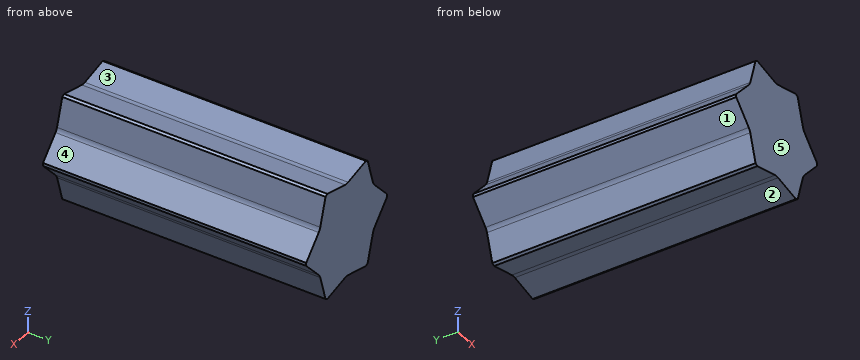
from build123d import *

# Parameters (mm, degrees)
EXTRUDE_1_DEPTH     = 1500
CUT_EXTRUDE_4_DEPTH = 1500
SHELL_START         = 10
SHELL_3_DEPTH       = 1480


# Read off the part's stored shape, not the designer's step: 抽壳3
with BuildPart() as part:
    # 草图2 → 凸台-拉伸1 (new body)
    with BuildSketch(Plane(origin=(0, 0, 0), x_dir=(1, 0, 0), z_dir=(0, 1, 0))):
        Polygon((345, 8.660254038), (180, 294.448637287), (165, 303.108891325), (-165, 303.108891325), (-180, 294.448637287), (-345, 8.660254038), (-345, -8.660254038), (-180, -294.448637287), (-165, -303.108891325), (165, -303.108891325), (180, -294.448637287), (345, -8.660254038), align=None)
    extrude(amount=EXTRUDE_1_DEPTH)

    # 草图5 → 切除-拉伸4 (cut)
    with BuildSketch(Plane(origin=(0, 0, 0), x_dir=(1, 0, 0), z_dir=(0, 1, 0))):
        with BuildLine():
            Line((238.21737139, 122.528375301), (345, 8.660254038))
            Line((345, 8.660254038), (379.520233023, 28.590519866))
            Line((379.520233023, 28.590519866), (334.34391274, 178.027059826))
            ThreePointArc((334.34391274, 178.027059826), (329.146090081, 190.032583711), (321.34791274, 200.536792121))
            Line((321.34791274, 200.536792121), (214.969297582, 314.638170659))
            Line((214.969297582, 314.638170659), (180, 294.448637287))
            Line((180, 294.448637287), (225.22137139, 145.038107596))
            ThreePointArc((225.22137139, 145.038107596), (230.419194049, 133.032583711), (238.21737139, 122.528375301))
        make_face()
        with BuildLine():
            Line((225.22137139, -145.038107596), (180, -294.448637287))
            Line((180, -294.448637287), (214.520233023, -314.378903115))
            Line((214.520233023, -314.378903115), (321.34791274, -200.536792121))
            ThreePointArc((321.34791274, -200.536792121), (329.146090081, -190.032583711), (334.34391274, -178.027059826))
            Line((334.34391274, -178.027059826), (379.969297582, -28.84978741))
            Line((379.969297582, -28.84978741), (345, -8.660254038))
            Line((345, -8.660254038), (238.21737139, -122.528375301))
            ThreePointArc((238.21737139, -122.528375301), (230.419194049, -133.032583711), (225.22137139, -145.038107596))
        make_face()
        with BuildLine():
            Line((12.996, 267.566482896), (165, 303.108891325))
            Line((165, 303.108891325), (165, 342.969422981))
            Line((165, 342.969422981), (12.996, 378.563851946))
            ThreePointArc((12.996, 378.563851946), (0, 380.065167421), (-12.996, 378.563851946))
            Line((-12.996, 378.563851946), (-165, 343.487958069))
            Line((-165, 343.487958069), (-165, 303.108891325))
            Line((-165, 303.108891325), (-12.996, 267.566482896))
            ThreePointArc((-12.996, 267.566482896), (0, 266.065167421), (12.996, 267.566482896))
        make_face()
        with BuildLine():
            Line((-12.996, -267.566482896), (-165, -303.108891325))
            Line((-165, -303.108891325), (-165, -342.969422981))
            Line((-165, -342.969422981), (-12.996, -378.563851946))
            ThreePointArc((-12.996, -378.563851946), (0, -380.065167421), (12.996, -378.563851946))
            Line((12.996, -378.563851946), (165, -343.487958069))
            Line((165, -343.487958069), (165, -303.108891325))
            Line((165, -303.108891325), (12.996, -267.566482896))
            ThreePointArc((12.996, -267.566482896), (0, -266.065167421), (-12.996, -267.566482896))
        make_face()
        with BuildLine():
            Line((-238.21737139, -122.528375301), (-345, -8.660254038))
            Line((-345, -8.660254038), (-379.520233023, -28.590519866))
            Line((-379.520233023, -28.590519866), (-334.34391274, -178.027059826))
            ThreePointArc((-334.34391274, -178.027059826), (-329.146090081, -190.032583711), (-321.34791274, -200.536792121))
            Line((-321.34791274, -200.536792121), (-214.969297582, -314.638170659))
            Line((-214.969297582, -314.638170659), (-180, -294.448637287))
            Line((-180, -294.448637287), (-225.22137139, -145.038107596))
            ThreePointArc((-225.22137139, -145.038107596), (-230.419194049, -133.032583711), (-238.21737139, -122.528375301))
        make_face()
        with BuildLine():
            Line((-225.22137139, 145.038107596), (-180, 294.448637287))
            Line((-180, 294.448637287), (-214.520233023, 314.378903115))
            Line((-214.520233023, 314.378903115), (-321.34791274, 200.536792121))
            ThreePointArc((-321.34791274, 200.536792121), (-329.14609008, 190.032583711), (-334.34391274, 178.027059826))
            Line((-334.34391274, 178.027059826), (-379.969297582, 28.84978741))
            Line((-379.969297582, 28.84978741), (-345, 8.660254038))
            Line((-345, 8.660254038), (-238.21737139, 122.528375301))
            ThreePointArc((-238.21737139, 122.528375301), (-230.419194049, 133.032583711), (-225.22137139, 145.038107596))
        make_face()
    extrude(amount=CUT_EXTRUDE_4_DEPTH, mode=Mode.SUBTRACT)

    # 抽壳3 outline → 抽壳3 (cut)
    with BuildSketch(Plane(origin=(0, 0, 0), x_dir=(1, 0, 0), z_dir=(0, 1, 0)).offset(SHELL_START)):
        with BuildLine():
            Line((-163.425407286, 292.470977468), (-171.574592714, 287.766043068))
            Line((-171.574592714, 287.766043068), (-215.64921864, 142.144339856))
            ThreePointArc((-215.64921864, 142.144339856), (-221.758128865, 128.033988697), (-230.922998431, 115.687897825))
            Line((-230.922998431, 115.687897825), (-335, 4.7049344))
            Line((-335, 4.7049344), (-335, -4.7049344))
            Line((-335, -4.7049344), (-230.92521864, -115.68553172))
            ThreePointArc((-230.92521864, -115.68553172), (-221.759751192, -128.031178744), (-215.650157642, -142.141234046))
            Line((-215.650157642, -142.141234046), (-171.574592714, -287.766043068))
            Line((-171.574592714, -287.766043068), (-163.425407286, -292.470977468))
            Line((-163.425407286, -292.470977468), (-15.276, -257.829871576))
            ThreePointArc((-15.276, -257.829871576), (-0.001622327, -256.065167441), (15.272840788, -257.829131872))
            Line((15.272840788, -257.829131872), (163.425407286, -292.470977468))
            Line((163.425407286, -292.470977468), (171.574592714, -287.766043068))
            Line((171.574592714, -287.766043068), (215.64921864, -142.144339856))
            ThreePointArc((215.64921864, -142.144339856), (221.758128865, -128.033988697), (230.922998431, -115.687897825))
            Line((230.922998431, -115.687897825), (335, -4.704934401))
            Line((335, -4.704934401), (335, 4.7049344))
            Line((335, 4.7049344), (230.92521864, 115.68553172))
            ThreePointArc((230.92521864, 115.68553172), (221.759751192, 128.031178744), (215.650157642, 142.141234046))
            Line((215.650157642, 142.141234046), (171.574592714, 287.766043068))
            Line((171.574592714, 287.766043068), (163.425407286, 292.470977468))
            Line((163.425407286, 292.470977468), (15.276, 257.829871576))
            ThreePointArc((15.276, 257.829871576), (0.001622327, 256.065167441), (-15.272840788, 257.829131872))
            Line((-15.272840788, 257.829131872), (-163.425407286, 292.470977468))
        make_face()
    extrude(amount=SHELL_3_DEPTH, mode=Mode.SUBTRACT)


solid = part.part
CAD build for the part. Positions are in the model's coordinates, mm. Face numbers are marked on the shaded views. A direction names the side the tool comes from. Round coordinates to 2 decimals unless told otherwise and drop trailing zeros. Loops run counter-clockwise (first coordinate to the right, second up) from the corner with the lowest first, then second, coordinate; pieces in that order, holes last.
(1) Wall check: line 1 along Y through (x, z) = (75, 202.5); line 2 along X through (y, z) = (1428, 0.5); line 3 along Z through (x, y) = (2, 109.5). Give the ranges that are in metal, low to high.
(2) Cut at B-B (z = -46). Give the cut face in (x, y).
(3) Drop flat-ended pins along their axis: pin 1 (12 mm diameter, centred on x = -259.5, y = 800, fed in from +Z); pin 2 (1.5 mm diameter, centred on x = -250.5, y = 679.5, fed in from +Z); pin 3 (2 mm diameter, centred on x = 255.5, y = 1285, fed in from -Z). Give the stop position or say it passes through.
(4) Which spindle directions (+Z, -Z, +X, -X, +Y, -Y) get a long thin tool onto all of the face, cutting with end or side? Do the marked faces 1 and 2. Say none if no direction does.
(5) Cut at A-A (x = 276.5). Give the cut face in (y, z), plus the area to 3 significant figures.
(6) Two-plate mould, pull along X, no slides. Class the marked faces 3, 4 and 5: +X half, -X half, draft (parallel to the pull), parting line (faces both ways), or undercut.
Findings below:
1. line 1: y = 0 to 10, 1490 to 1500
1. line 2: x = -345 to -335, 335 to 345
1. line 3: z = -266.1 to -256.1, 256.1 to 266.1
2. outline: (-309.98, 0) - (309.98, 0) - (309.98, 1500) - (-309.98, 1500) - close; hole (-296.27, 10) - (296.27, 10) - (296.27, 1490) - (-296.27, 1490) - close
3. pin 1: stops at z = 106.23
3. pin 2: stops at z = 110.23
3. pin 3: stops at z = -105.17
4. face 1: -Z, -X, +Y, -Y
4. face 2: -Z, +Y, -Y
5. outline: (0, -81.71) - (1500, -81.71) - (1500, 81.71) - (0, 81.71) - close; hole (10, -67.09) - (1490, -67.09) - (1490, 67.09) - (10, 67.09) - close
5. area: 46,500 mm2
6. face 3: undercut
6. face 4: +X half
6. face 5: draft
